Work out the finished part from the listing and answer in its coordinate system (mm). Face numbers are marked on the shaded views. A direction names the side the tool comes from. Round coordinates to 2 decimals unless told otherwise and drop trailing zeros. Order: outer loops, then holes, each group sorted by start corner. A loop starts at its lowest first (then second) coordinate and runs counter-clockwise, first axis right, second up.
from build123d import *

# Parameters (mm, degrees)
SKETCH_1_R          = 6
EXTRUDE_1_DEPTH     = 11
EXTRUDE_2_DEPTH     = 3
EXTRUDE_3_DEPTH     = 3
SKETCH_5_R          = 6
EXTRUDE_4_DEPTH     = 10
SKETCH_6_R          = 1.5
CUT_EXTRUDE_1_DEPTH = 32.717503054
CUT_EXTRUDE_START   = -2.5
SKETCH_7_R          = 6
SKETCH_7_R_2        = 5.5
CUT_EXTRUDE_2_DEPTH = 2.5
SKETCH_8_R          = 1
CUT_EXTRUDE_3_DEPTH = 28.586228448
SKETCH_9_R          = 2.75
CUT_EXTRUDE_4_DEPTH = 5


with BuildPart() as part:
    # 草图1 → 凸台-拉伸1 (new body)
    with BuildSketch(Plane.XY):
        Circle(SKETCH_1_R)
    extrude(amount=EXTRUDE_1_DEPTH)

    # 草图2 → 凸台-拉伸2 (add)
    with BuildSketch(Plane.XY):
        with BuildLine():
            Line((-19, 4), (19, 4))
            ThreePointArc((19, 4), (23, 0), (19, -4))
            Line((19, -4), (-19, -4))
            ThreePointArc((-19, -4), (-23, 0), (-19, 4))
        make_face()
    extrude(amount=EXTRUDE_2_DEPTH)

    # 草图3 → 凸台-拉伸3 (add)
    with BuildSketch(Plane.XY.offset(11)):
        with BuildLine():
            Line((-19, 4), (19, 4))
            ThreePointArc((19, 4), (23, 0), (19, -4))
            Line((19, -4), (-19, -4))
            ThreePointArc((-19, -4), (-23, 0), (-19, 4))
        make_face()
    extrude(amount=EXTRUDE_3_DEPTH)

    # 草图5 → 凸台-拉伸4 (add)
    with BuildSketch(Plane.XY.offset(11)):
        with Locations(Location((0, 0, 0), (0, 0, 221.810314896))):
            Circle(SKETCH_5_R)
    extrude(amount=EXTRUDE_4_DEPTH)

    # 草图6 → 切除-拉伸1 (cut, through all)
    with BuildSketch(Plane(origin=(0, 0, 0), x_dir=(-1, 0, 0), z_dir=(0, 0, -1))):
        Circle(SKETCH_6_R)
    extrude(amount=-CUT_EXTRUDE_1_DEPTH, mode=Mode.SUBTRACT)

    # 草图7 → 切除-拉伸2 (cut)
    with BuildSketch(Plane.XY.offset(21).offset(CUT_EXTRUDE_START)):
        with Locations(Location((0, 0, 0), (0, 0, 221.810314896))):
            Circle(SKETCH_7_R)
        Circle(SKETCH_7_R_2, mode=Mode.SUBTRACT)
    extrude(amount=CUT_EXTRUDE_2_DEPTH, mode=Mode.SUBTRACT)

    # 草图8 → 切除-拉伸3 (cut, through all)
    with BuildSketch(Plane.XY.offset(14)):
        with Locations((-19, 0)):
            Circle(SKETCH_8_R)
        with Locations((19, 0)):
            Circle(SKETCH_8_R)
    extrude(amount=-CUT_EXTRUDE_3_DEPTH, mode=Mode.SUBTRACT)

    # 草图9 → 切除-拉伸4 (cut)
    with BuildSketch(Plane.XY.offset(21)):
        Circle(SKETCH_9_R)
    extrude(amount=-CUT_EXTRUDE_4_DEPTH, mode=Mode.SUBTRACT)


solid = part.part
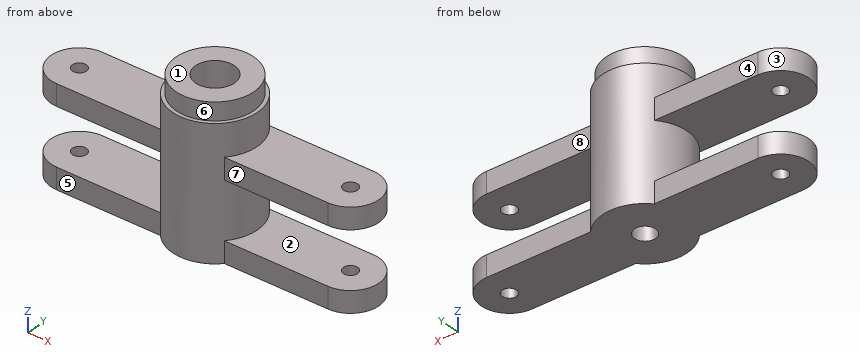
Item 1: A tool of negligible diameter and unlimited length cuts with its end or side. For the marked faces 4, 5, 6, 7 and 8, from which of +Z, -Z, +X, -X, +Y, -Y can it reach the whole face along a straight path? Write none if from no direction.
Item 2: Find section C-C (y = 0). State how many separate pieces and enclosed holes the cut face has, plus the area to 3 significant figures.
Item 3: Find section A-A (x = 0). Write down the section's boundary in (y, z).
Item 4: Given pin 1 (5 mm diameter, centred on x = 18, z = 15.5, fed in from +Y); pin 2 (1.5 mm diameter, centred on y = 3, z = 8, fed in from -X); pin 3 (0.9 mm diameter, centred on x = 8.5, z = 12.5, fed in from -Y), each flat-ended and moving along its own axis, determine where each tip first touches the part or whether it passes through.
Item 5: Find the intervals of material crossed by line 1 along Z through (x, y) = (20, 2.5); line 2 along Y through (x, z) = (19, 12.35); line 3 along X through (y, z) = (4, 6), in increasing order.
Item 6: Find section D-D (z = 8). Write down the section's boundary in (x, y), plus the area to 3 significant figures.
Item 7: For a pull along Z with two mould halves and no side action, classify the marked faces 1, 2 and 3 as released by +Z, released by -Z, zero draft, split by the parting line, or undercut.
Item 8: Find section B-B (x = -13). Write down the section's boundary in (y, z), plus the area to 3 significant figures.
Model answer:
1. face 4: +Z, -Z, -X, +Y
1. face 5: +Z, -Z, -X, -Y
1. face 6: +Z
1. face 7: +Z, -Z, +X, -Y
1. face 8: +Z, -Z, +X, +Y
2. separate pieces: 6
2. enclosed holes: 0
2. area: 354 mm2
3. outline: (-6, 0) - (-1.5, 0) - (-1.5, 16) - (-2.75, 16) - (-2.75, 21) - (-5.5, 21) - (-5.5, 18.5) - (-6, 18.5) - close; (1.5, 0) - (6, 0) - (6, 18.5) - (5.5, 18.5) - (5.5, 21) - (2.75, 21) - (2.75, 16) - (1.5, 16) - close
4. pin 1: stops at y = 4
4. pin 2: stops at x = -5.56
4. pin 3: stops at y = -4
5. line 1: z = 0 to 3, 11 to 14
5. line 2: y = -4 to -1, 1 to 4
5. line 3: x = -4.47 to 4.47
6. outline: circle Ø12 at (0, 0); hole circle Ø3 at (0, 0)
6. area: 106 mm2
7. face 1: released by +Z
7. face 2: undercut
7. face 3: zero draft
8. outline: (-4, 0) - (4, 0) - (4, 3) - (-4, 3) - close; (-4, 11) - (4, 11) - (4, 14) - (-4, 14) - close
8. area: 48.0 mm2
